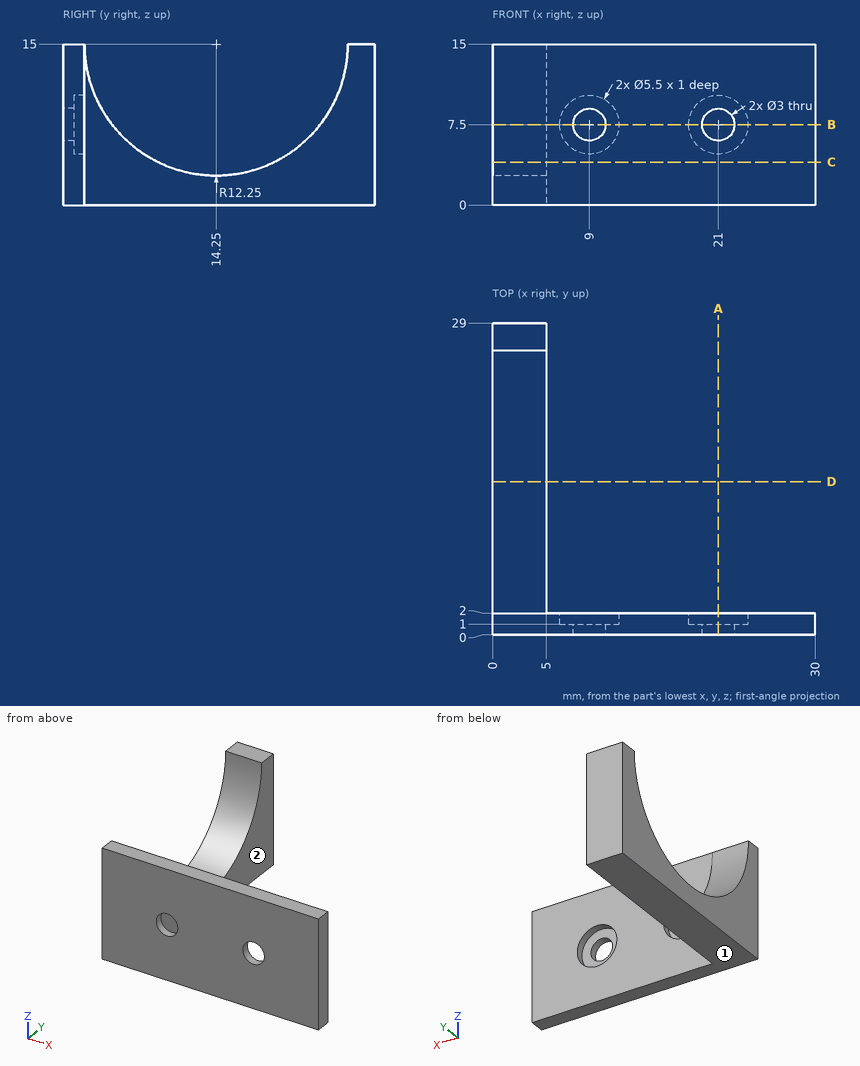
The figure shows three views and two pictorial views of one solid part (mm, origin at its lowest corner). Answer the questions. A direction names the side the tool comes from. Round coordinates to 2 decimals unless told otherwise and drop trailing zeros. Order: outer loops, then holes, each group sorted by start corner. A loop starts at its lowest first (then second) coordinate and runs counter-clockwise, first axis right, second up. Notation, with made-up numbers: M -10.5,58.5 L 29.5,58.5 A23 ccw 29.5,90.5 Z; hole C 5.25,46 d9. An arc over 180 degrees is marked long. Put each result on its own line as item: value. Start each with the question number.
Q1. Straight lines are drawn through the part: L1, parallel to Z at x = 9, y = 1.4; L2, parallel to Z at x = 9, y = 0.65; L3, parallel to X at y = 27, z = 5.5. For each, find the intervals that lie inside material, in ascending order. Write a range as [from, to].
Q2. Section C-C, the plane z = 4 is taken. Write down the section's boundary in (x, y).
Q3. Section A-A, the plane x = 21 is taken. Write down the section's boundary in (y, z).
Q4. Flat-ended cylindrical pins translate along their axes: pin 1 (6.5 mm diameter, centred on x = 21, z = 7.5, fed in from +Y); pin 2 (1.5 mm diameter, centred on y = 23.5, z = 5, fed in from +X); pin 3 (4 mm diameter, centred on x = 9, z = 7.5, fed in from +Y). Find the tip coordinate at first contact, or state that the pin passes through.
Q5. Section B-B, the plane z = 7.5 is taken. Write down the section's boundary in (x, y), and give its area (3 significant figures).
Q6. A tool of negligible diameter and unlimited length cuts with its end or side. For the marked faces 1 and 2, from which of +Z, -Z, +X, -X, +Y, -Y can it reach the whole face along a straight path? Write none if from no direction.
Q7. Section D-D, the plane y = 14.25 is taken. Write down the section's boundary in (x, z), and give its area (4 significant figures).
Findings below:
1. L1: z = [0, 4.75], [10.25, 15]
1. L2: z = [0, 6], [9, 15]
1. L3: x = [0, 5]
2. outline: M 0,0 L 30,0 L 30,2 L 5,2 L 5,8.86 L 0,8.86 Z; M 0,19.64 L 5,19.64 L 5,29 L 0,29 Z
3. outline: M 0,0 L 2,0 L 2,4.75 L 1,4.75 L 1,6 L 0,6 Z; M 0,9 L 1,9 L 1,10.25 L 2,10.25 L 2,15 L 0,15 Z
4. pin 1: stops at y = 2
4. pin 2: stops at x = 5
4. pin 3: stops at y = 1
5. outline: M 0,0 L 7.5,0 L 7.5,1 L 6.25,1 L 6.25,2 L 5,2 L 5,4.56 L 0,4.56 Z; M 0,23.94 L 5,23.94 L 5,29 L 0,29 Z; M 10.5,0 L 19.5,0 L 19.5,1 L 18.25,1 L 18.25,2 L 11.75,2 L 11.75,1 L 10.5,1 Z; M 22.5,0 L 30,0 L 30,2 L 23.75,2 L 23.75,1 L 22.5,1 Z
5. area: 81.1 mm^2
6. face 1: -Z, +X, -X, +Y, -Y
6. face 2: +Z, -Z, +X, +Y
7. outline: M 0,0 L 5,0 L 5,2.75 L 0,2.75 Z
7. area: 13.75 mm^2
